Autodesk Inventor part; units mm, degrees
ref_plane "Work Plane4" through (44, 12.5, 0) normal (0, 1, 0) x (-1, 0, 0)
ref_plane "Work Plane6" through (0, 4.75, 0) normal (0, 1, 0) x (-1, 0, 0)
ref_plane "YZ Plane" through (0, 0, 0) normal (1, 0, 0) x (0, 1, 0)
sketch "Sketch1" plane through (0, 0, 0) normal (0, 0, 1) x (1, 0, 0)
  line L0 (0, 0) -> (239, 0)
  line L1 (239, 0) -> (239, 9.5)
  line L2 (0, 0) -> (0, 12.5)
  line L3 (0, 12.5) -> (88, 12.5)
  line L4 (239, 9.5) -> (88, 9.5)
  line L5 (88, 9.5) -> (88, 12.5)
  dimension "d1" = 9.5
  dimension "d3" = 12.5
  dimension "d19" = 88
  dimension "d21" = 151
revolve "Revolution1" add sketch "Sketch1" angle 360 about axis through (0, 0, 0) along (1, 0, 0)
ref_plane "Work Plane3" through (44, 12.5, 0) normal (0, 1, 0) x (-1, 0, 0)
ref_plane "Work Plane4" through (44, 12.5, 0) normal (0, 1, 0) x (-1, 0, 0)
ref_plane "Work Plane5" through (163.5, 9.5, 0) normal (0, 1, 0) x (-1, 0, 0)
sketch "Sketch6" plane through (163.5, 9.5, 0) normal (0, 1, 0) x (-1, 0, 0)
  line L0 (-75.5, 9.5) -> (-75.5, -9.5)
  circle A0 centre (-64.5, 0) radius 5
  point P0 (163.5, 0)
  point P1 (-75.5, 0)
  dimension "d27" = 10
  dimension "d28" = 11
extrude "Extrusion5" cut sketch "Sketch6" against normal blind 2
sketch "Sketch7" plane through (228, 7.5, 0) normal (0, 1, 0) x (1, 0, 0)
  circle A0 centre (0, 0) radius 2
  point P0 (-228, 0)
  dimension "d32" = 4
extrude "Extrusion6" cut sketch "Sketch7" against normal blind 5
fillet "Fillet2" radius 3.5 1 edges at (226, 7.5, 0)
sketch "Sketch8" plane through (44, 12.5, 0) normal (0, 1, 0) x (-1, 0, 0)
  point P0 (44, 0)
sketch "Sketch9" plane through (163.5, 9.5, 0) normal (0, 1, 0) x (-1, 0, 0)
  circle A0 centre (-64.5, 0) radius 5
  line L0 (-64.5, 5) -> (-56.5, 5)
  line L1 (-64.5, -5) -> (-56.5, -5)
  line L2 (-56.5, -5) -> (-56.5, 5)
  point P0 (163.5, 0)
  dimension "d36" = 8
  dimension "d37" = 8
extrude "Extrusion7" cut sketch "Sketch9" against normal blind 2 contours A0 L0 L2 L1
ref_plane "Work Plane6" through (0, 4.75, 0) normal (0, 1, 0) x (-1, 0, 0)
properties part number "eixo final"
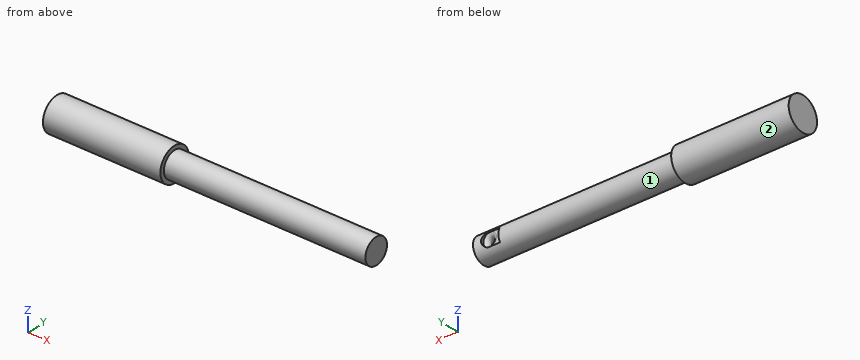
Geometry: final body of the model. Coordinates: model frame, mm. Face numbers are marked on the shaded views. A direction names the side the tool comes from. Coordinates: 2 decimals unless noted, no trailing zeros. Write each loop counter-clockwise with the first axis right and the second up, starting at its lowest first coordinate (ties: lowest second). Pieces come first, ordered by that corner, then holes. Notation, with made-up numbers: M -21.5,-33.5 L -0.5,-33.5 A26 ccw -0.5,-19.5 Z; hole C 11.25,52 d11. An arc over 180 degrees is marked long. Use CSV: the item, a comma, the result in double quotes. Start each with the question number.
1. Cut plane C-C on x = 201.5. Return the cut outline in (y, z).
2. Reachability of the marked faces 1 and 2 from +Z, -Z, +X, -X, +Y, -Y: full face, straight path, thin tool, end or side. Return the list, or none.
3. Cut plane A-A on y = 0. Return the cut outline in (x, z).
4. Cut plane D-D on x = 30. Return the cut outline in (y, z).
5. First-contact query: P1, Ø0.5, axis at x = 225.5, y = 8, coming from the +Z side; P2, Ø10, axis at x = 145, y = 4.5, coming from the -Z side; P3, Ø0.5, axis at x = 224.5, y = 7.5, coming from the -Z side. Flat tips, straight axial feed; report the tip coordinate or a pass-through.
6. Cut plane B-B on z = 0. Return the cut outline in (x, y).
7. Ray query, probe 1 along X at (y, z) = (3.35, 0); probe 2 along Z at (x, y) = (228, 3.25); probe 3 along Y at (x, z) = (14, 0.25). Return the intervals inside material, ascending.
Entries:
1,outline,"C 0,0 d19"
2,face 1,"+X"
2,face 2,"+X, -X"
3,outline,"M 0,-12.5 L 88,-12.5 L 88,-9.5 L 239,-9.5 L 239,9.5 L 88,9.5 L 88,12.5 L 0,12.5 Z"
4,outline,"C 0,0 d25"
5,P1,"z = 5.49"
5,P2,"z = -9.5"
5,P3,"z = -6.14"
6,outline,"M 0,-12.5 L 88,-12.5 L 88,-9.5 L 239,-9.5 L 239,9.5 L 233,9.5 L 233,7.5 A3.5 ccw 230,4.04 L 230,2.5 L 226,2.5 L 226,4.04 A3.5 ccw 223,7.5 L 220,7.5 L 220,9.5 L 88,9.5 L 88,12.5 L 0,12.5 Z"
7,probe 1,"0 to 226, 230 to 239"
7,probe 2,"-8.93 to -2, 2 to 8.93"
7,probe 3,"-12.5 to 12.5"
